Autodesk Inventor part; units mm, degrees
ref_plane "YZ Plane" through (0, 0, 0) normal (1, 0, 0) x (0, 1, 0)
ref_plane "XZ Plane" through (0, 0, 0) normal (0, 1, 0) x (-1, 0, 0)
ref_plane "XY Plane" through (0, 0, 0) normal (0, 0, 1) x (1, 0, 0)
sketch "Sketch1" plane through (0, 0, 0) normal (0, 1, 0) x (-1, 0, 0)
  line L0 (-7, 5.75) -> (7, 5.75)
  line L1 (7, 5.75) -> (7, -5.75)
  line L2 (7, -5.75) -> (-7, -5.75)
  line L3 (-7, -5.75) -> (-7, 5.75)
  line L4 (7, 5.75) -> (-7, -5.75) construction
  line L5 (-7, -5.75) -> (-5.8, -5.75)
  line L6 (-7, -4.55) -> (-7, -5.75)
  line L7 (7, 5.75) -> (5.8, 5.75)
  line L8 (7, 4.55) -> (7, 5.75)
  circle A0 centre (-5.8, -4.55) radius 0.7
  circle A1 centre (5.8, 4.55) radius 0.7
  line L9 (-3, 3) -> (3, 3)
  line L10 (3, 3) -> (3, -3)
  line L11 (3, -3) -> (-3, -3)
  line L12 (-3, -3) -> (-3, 3)
  line L13 (-3, 3) -> (3, -3) construction
  line L14 (3, 3) -> (-3, -3) construction
  circle A2 centre (0.5, -0.45) radius 1.885
  point P0 (3.3, -2.75)
  point P1 (0, 0)
  dimension "d0" = 14
  dimension "d1" = 11.5
  dimension "d6" = 1.4
  dimension "d7" = 1.4
  dimension "d12" = 6
  dimension "d13" = 6
  dimension "d17" = 3.77
sketch "Sketch2" plane through (0, 0, 0) normal (0, 1, 0) x (-1, 0, 0)
  line L0 (-7, 5.75) -> (7, 5.75)
  line L1 (7, 5.75) -> (7, -5.75)
  line L2 (7, -5.75) -> (-7, -5.75)
  line L3 (-7, -5.75) -> (-7, 5.75)
  line L4 (7, 5.75) -> (-7, -5.75) construction
  line L5 (-7, -5.75) -> (-5.8, -5.75)
  line L6 (-7, -4.55) -> (-7, -5.75)
  line L7 (7, 5.75) -> (5.8, 5.75)
  line L8 (7, 4.55) -> (7, 5.75)
  circle A0 centre (-5.8, -4.55) radius 0.7
  circle A1 centre (5.8, 4.55) radius 0.7
  line L9 (-3, 3) -> (3, 3)
  line L10 (3, 3) -> (3, -3)
  line L11 (3, -3) -> (-3, -3)
  line L12 (-3, -3) -> (-3, 3)
  line L13 (-3, 3) -> (3, -3) construction
  line L14 (3, 3) -> (-3, -3) construction
  circle A2 centre (0.5, -0.45) radius 1.885
  point P0 (0, 0)
  point P1 (3.3, -2.75)
  point P2 (0, 0)
  dimension "d18" = 14
  dimension "d19" = 11.5
  dimension "d20" = 1.4
  dimension "d21" = 1.4
  dimension "d22" = 6
  dimension "d23" = 6
  dimension "d24" = 3.77
sketch "Sketch3" plane through (0, 0, 0) normal (0, 1, 0) x (-1, 0, 0)
  line L0 (-7, 5.75) -> (7, 5.75)
  line L1 (7, 5.75) -> (7, -5.75)
  line L2 (7, -5.75) -> (-7, -5.75)
  line L3 (-7, -5.75) -> (-7, 5.75)
  line L4 (7, 5.75) -> (-7, -5.75) construction
  line L5 (-7, -5.75) -> (-5.8, -5.75)
  line L6 (-7, -4.55) -> (-7, -5.75)
  line L7 (7, 5.75) -> (5.8, 5.75)
  line L8 (7, 4.55) -> (7, 5.75)
  circle A0 centre (-5.8, -4.55) radius 0.7
  circle A1 centre (5.8, 4.55) radius 0.7
  line L9 (-3, 3) -> (3, 3)
  line L10 (3, 3) -> (3, -3)
  line L11 (3, -3) -> (-3, -3)
  line L12 (-3, -3) -> (-3, 3)
  line L13 (-3, 3) -> (3, -3) construction
  line L14 (3, 3) -> (-3, -3) construction
  circle A2 centre (0.5, -0.45) radius 1.885
  point P0 (0, 0)
  point P1 (3.3, -2.75)
  point P2 (0, 0)
  dimension "d25" = 14
  dimension "d26" = 11.5
  dimension "d27" = 1.4
  dimension "d28" = 1.4
  dimension "d29" = 6
  dimension "d30" = 6
  dimension "d31" = 3.77
extrude "Extrusion1" add sketch "Sketch1" against normal blind 1 contours L0 L1 L2 L3 | L9 L10 L11 L12 | A2
extrude "Extrusion2" add sketch "Sketch2" along normal blind 2.1 contours L9 L10 L11 L12 | A2
extrude "Extrusion3" add sketch "Sketch3" along normal blind 0.7 from surface at 2.1 contours A2
sketch "Sketch4" plane through (0, -1, 0) normal (0, -1, 0) x (1, 0, 0)
  line L0 (3, -3) -> (-3, -3)
  line L1 (-3, -3) -> (-3, 3)
  line L2 (-3, 3) -> (3, 3)
  line L3 (3, 3) -> (3, -3)
  line L4 (3, -3) -> (-3, 3) construction
  line L5 (-3, -3) -> (3, 3) construction
  point P0 (0, 0)
  dimension "d38" = 6
  dimension "d39" = 6
extrude "Extrusion4" add sketch "Sketch4" along normal blind 1
properties part number "optical"
Could you check a few things on this model? Use its own coordinates, in mm. A direction names the side the tool comes from. Give positions to 0.01 mm unless a question says otherwise; leave off trailing zeros. Order: outer loops, then holes, each group sorted by start corner. A loop starts at its lowest first (then second) coordinate and runs counter-clockwise, first axis right, second up. Notation, with made-up numbers: (0, 58.25) - (49, 58.25) arc R32 ccw to (49, 97.25) - close; hole circle Ø2 at (5, -9). An arc over 180 degrees is marked (long way). One line per item, written item: value. Start each with the question number.
1. Imagine slicing it at B-B on x = 5.8. List the corners of the cut face in (y, z) for me.
2. Imagine slicing it at A-A on z = -4.55. List the corners of the cut face in (x, y) for me, plus the area to 3 significant figures.
3. For P1, Ø1.3, axis at x = 5.8, z = -4.55, coming from the -Y side; P2, Ø0.6, axis at x = 1, y = 0.5, coming from the -Z side; P3, Ø1.8, axis at x = -5.8, z = 4.55, coming from the -Y side; P4, Ø2.5, axis at y = 1.5, z = 0.5, coming from the -X side, each with a flat end and sliding along its axis, tell me the tip position at first contact or that it passes through.
4. Imagine slicing it at D-D on x = -2.75. List the corners of the cut face in (y, z) for me.
5. For faces 1 (the face through (0, -1.5, -3)), 2 (the face through (0, 1, 3)), 3 (the face through (1, 2.1, 1)), 4 (the face through (0, -1.5, 3)), which set-ups out of +Z, -Z, +X, -X, +Y, -Y let a thin tool reach every point of the face, with its end or its side?
6. Thinking about a two-plate mould opening in X: for faces 5 (the face through (6.32, -0.49, -4.08)), 6 (the face through (3, -1.5, 0)), 7 (the face through (0, 1, -3)), which applies, +X half, -X half, draft (parallel to the pull), parting line (faces both ways), or undercut?
7. If I drill on probe 1 along Z at (x, y) = (-5.8, -0.4); probe 2 along X at (y, z) = (-1.05, 1); probe 3 along Y at (x, z) = (2.5, 4), over which ranges is the centre line in solid material (lowest first)?
8. Imagine slicing it at C-C on y = -0.4. List the corners of the cut face in (x, z) for me, plus the area to 3 significant figures.
Values:
1. outline: (-1, -5.75) - (0, -5.75) - (0, -5.25) - (-1, -5.25) - close; (-1, -3.85) - (0, -3.85) - (0, 5.75) - (-1, 5.75) - close
2. outline: (-7, -1) - (5.1, -1) - (5.1, 0) - (-7, 0) - close; (6.5, -1) - (7, -1) - (7, 0) - (6.5, 0) - close
2. area: 12.6 mm²
3. P1: through
3. P2: z = -3
3. P3: y = -1
3. P4: x = -3
4. outline: (-2, -3) - (-1, -3) - (-1, -5.75) - (0, -5.75) - (0, -3) - (2.1, -3) - (2.1, 3) - (0, 3) - (0, 5.75) - (-1, 5.75) - (-1, 3) - (-2, 3) - close
5. face 1: -Z, +X, -X, -Y
5. face 2: +Z, +X, -X, +Y
5. face 3: +Y
5. face 4: +Z, +X, -X, -Y
6. face 5: undercut
6. face 6: +X half
6. face 7: draft
7. probe 1: -5.75 to 3.85, 5.25 to 5.75
7. probe 2: -3 to 3
7. probe 3: -1 to 0
8. outline: (-7, -5.75) - (7, -5.75) - (7, 5.75) - (-7, 5.75) - close; hole circle Ø1.4 at (-5.8, 4.55); hole circle Ø1.4 at (5.8, -4.55)
8. area: 158 mm²
